The model under review builds one solid part; all positions refer to its coordinate system, in mm. A direction names the side the tool comes from. Give positions to 0.01 mm unless a question says otherwise; leave off trailing zeros. Loops run counter-clockwise (first coordinate to the right, second up) from the corner with the lowest first, then second, coordinate; pieces in that order, holes last. Notation, with made-up numbers: M 23,80 L 55,80 A18 ccw 55,101 Z; hole C 62,-36.5 d8. An arc over 180 degrees is marked long. Put each result on its own line as item: value. Start each with the question number.
```python
from build123d import *

# Parameters (mm, degrees)
SM_BASE_FLANGE_1_DEPTH = 133
CUT_EXTRUDE_1_REACH    = 149.557
SKETCH_2_R             = 1
SKETCH_2_R_2           = 11.5
M3X0_5_1_D             = 2.5
M3X0_5_1_DEPTH         = 7.5
M3X0_5_1_CBORE_D       = 3
M3X0_5_1_CBORE_DEPTH   = 6
M3X0_5_1_TIP           = 0.751075774
SKETCH_5_R             = 2.25
CUT_EXTRUDE_2_DEPTH    = 148.271857461


# Sheet-metal steps are written as plain solids
with BuildPart() as part:
    # Sketch 1 → 基材-凸緣1 (new body)
    with BuildSketch(Plane.XY):
        with BuildLine():
            Line((0, 60), (0, 0.7366))
            ThreePointArc((0, 0.7366), (0.215745145, 0.215745145), (0.7366, 0))
            Line((0.7366, 0), (20, 0))
            Line((20, 0), (20, -2))
            Line((20, -2), (0.7366, -2))
            ThreePointArc((0.7366, -2), (-1.198468417, -1.198468417), (-2, 0.7366))
            Line((-2, 0.7366), (-2, 60))
            Line((-2, 60), (0, 60))
        make_face()
    extrude(amount=SM_BASE_FLANGE_1_DEPTH)

    # Sketch 2 → 除料-伸長1 (cut, up to next)
    with BuildSketch(Plane.ZY.offset(2), mode=Mode.PRIVATE) as cut_extrude_1_sk1:
        with Locations((103, 39)):
            Circle(SKETCH_2_R)
    cut_extrude_1_tool1 = extrude(cut_extrude_1_sk1.sketch, amount=-CUT_EXTRUDE_1_REACH, mode=Mode.PRIVATE) & part.part
    # Sketch 2 → 除料-伸長1 (cut, up to next)
    with BuildSketch(Plane.ZY.offset(2), mode=Mode.PRIVATE) as cut_extrude_1_sk2:
        with Locations((54, 39)):
            Circle(SKETCH_2_R)
    cut_extrude_1_tool2 = extrude(cut_extrude_1_sk2.sketch, amount=-CUT_EXTRUDE_1_REACH, mode=Mode.PRIVATE) & part.part
    # Sketch 2 → 除料-伸長1 (cut, up to next)
    with BuildSketch(Plane.ZY.offset(2), mode=Mode.PRIVATE) as cut_extrude_1_sk3:
        with Locations((54, 35)):
            Circle(SKETCH_2_R)
    cut_extrude_1_tool3 = extrude(cut_extrude_1_sk3.sketch, amount=-CUT_EXTRUDE_1_REACH, mode=Mode.PRIVATE) & part.part
    # Sketch 2 → 除料-伸長1 (cut, up to next)
    with BuildSketch(Plane.ZY.offset(2), mode=Mode.PRIVATE) as cut_extrude_1_sk4:
        with Locations((20, 37)):
            Circle(SKETCH_2_R_2)
    cut_extrude_1_tool4 = extrude(cut_extrude_1_sk4.sketch, amount=-CUT_EXTRUDE_1_REACH, mode=Mode.PRIVATE) & part.part
    add(cut_extrude_1_tool1.solids().sort_by_distance((-2, 39, 103))[0], mode=Mode.SUBTRACT)
    add(cut_extrude_1_tool2.solids().sort_by_distance((-2, 39, 54))[0], mode=Mode.SUBTRACT)
    add(cut_extrude_1_tool3.solids().sort_by_distance((-2, 35, 54))[0], mode=Mode.SUBTRACT)
    add(cut_extrude_1_tool4.solids().sort_by_distance((-2, 37, 20))[0], mode=Mode.SUBTRACT)

    # M3x0.5 螺紋孔1
    with Locations(Plane.ZY.offset(2)):
        with Locations((32.5, 49.5), (32.5, 24.5), (7.5, 49.5), (7.5, 24.5)):
            CounterBoreHole(M3X0_5_1_D / 2, M3X0_5_1_CBORE_D / 2, M3X0_5_1_CBORE_DEPTH, depth=M3X0_5_1_DEPTH)
            with Locations((0, 0, -(M3X0_5_1_DEPTH + M3X0_5_1_TIP / 2))):  # 118° drill point
                Cone(0, M3X0_5_1_D / 2, M3X0_5_1_TIP, mode=Mode.SUBTRACT)

    # 草圖5 → 除料-伸長2 (cut, through all)
    with BuildSketch(Plane(origin=(0, 0, 0), x_dir=(1, 0, 0), z_dir=(0, 1, 0))):
        with Locations(Location((11.5, -125, 0), (0, 0, 270))):
            Circle(SKETCH_5_R)
        with Locations(Location((11.5, -80, 0), (0, 0, 270))):
            Circle(SKETCH_5_R)
        with Locations(Location((11.5, -53, 0), (0, 0, 270))):
            Circle(SKETCH_5_R)
        with Locations(Location((11.5, -8, 0), (0, 0, 270))):
            Circle(SKETCH_5_R)
    extrude(amount=-CUT_EXTRUDE_2_DEPTH, mode=Mode.SUBTRACT)


solid = part.part
```
Item 1: Consider section D-D, the plane z = 35.5. Write out the cut boundary in (x, y).
Item 2: Consider section C-C, the plane y = 31. Write out the cut boundary in (x, z).
Item 3: Clearance check with flat-ended pins moving along their axes: pin 1 Ø2.5 at (y, z) = (49.5, 32.5) entering from +X; pin 2 Ø2.5 at (y, z) = (39, 103) entering from +X; pin 3 Ø9.5 at (x, z) = (10, 46) entering from +Y. State where each tip first meets the part, or that it passes through.
Item 4: Consider section A-A, the plane z = 80. Write out the cut boundary in (x, y).
Item 5: Draft analysis for pull direction Z (two halves, no side actions). For faces 3 (the cylindrical face through (12.176, -0.986, 127.146)), 4 (the flat face through (11, -2, 66)), 5 (the flat face through (-1, 20, 133)), 6 (the cylindrical face through (12.176, -0.986, 82.146)), state which applies: +Z half, -Z half, draft (parallel to the pull), parting line (faces both ways), or undercut.
Item 6: Consider section B-B, the plane x = 11.5. Write out the cut boundary in (y, z), plus the area to 3 significant figures.
Item 7: To check wall thickness, follow L1, parallel to Y at x = -0.8, z = 32.5; L2, parallel to Y at x = -0.45, z = 32.5; L3, parallel to X at y = 19, z = 69. State the ranges of each line that lie inside material, in increasing order. Write a range as [from, to].
Item 8: Tool access review of faces 1 (the flat face through (-2, 30, 66)), 2 (the flat face through (10, 0, 66)): name each direction out of +Z, -Z, +X, -X, +Y, -Y from which nothing blocks a thin tool from reaching the whole face with its end or side.
Report:
1. outline: M -2,0.74 A2.74 ccw 0.74,-2 L 20,-2 L 20,0 L 0.74,0 A0.74 cw 0,0.74 L 0,60 L -2,60 Z
2. outline: M -2,0 L 0,0 L 0,10.19 L -2,10.19 Z; M -2,29.81 L 0,29.81 L 0,133 L -2,133 Z
3. pin 1: through
3. pin 2: x = 0
3. pin 3: y = 0
4. outline: M -2,0.74 A2.74 ccw 0.74,-2 L 9.25,-2 L 9.25,0 L 0.74,0 A0.74 cw 0,0.74 L 0,60 L -2,60 Z; M 13.75,-2 L 20,-2 L 20,0 L 13.75,0 Z
5. face 3: undercut
5. face 4: draft
5. face 5: +Z half
5. face 6: undercut
6. outline: M -2,0 L 0,0 L 0,5.75 L -2,5.75 Z; M -2,10.25 L 0,10.25 L 0,50.75 L -2,50.75 Z; M -2,55.25 L 0,55.25 L 0,77.75 L -2,77.75 Z; M -2,82.25 L 0,82.25 L 0,122.75 L -2,122.75 Z; M -2,127.25 L 0,127.25 L 0,133 L -2,133 Z
6. area: 230 mm²
7. L1: [-1.53, 23], [26, 48], [51, 60]
7. L2: [-1.73, 23], [26, 48], [51, 60]
7. L3: [-2, 0]
8. face 1: +Z, -Z, -X, +Y, -Y
8. face 2: +Z, -Z, +X, +Y
